```python
from build123d import *

# Parameters (mm, degrees)
SKETCH1_R            = 10
SKETCH1_R_2          = 5
BOSS_EXTRUDE1_DEPTH  = 10
SKETCH2_R            = 7
SKETCH2_R_2          = 5
BOSS_EXTRUDE2_DEPTH  = 3.5
SKETCH3_R            = 10
SKETCH3_R_2          = 5
BOSS_EXTRUDE3_DEPTH  = 10
SKETCH4_R            = 7
SKETCH4_R_2          = 5
BOSS_EXTRUDE4_DEPTH  = 3.5
SKETCH5_R            = 10
SKETCH5_R_2          = 5
BOSS_EXTRUDE5_DEPTH  = 10
SKETCH6_R            = 7
SKETCH6_R_2          = 5
BOSS_EXTRUDE6_DEPTH  = 3.5
SKETCH7_R            = 10
SKETCH7_R_2          = 5
BOSS_EXTRUDE7_DEPTH  = 10
SKETCH8_R            = 7
SKETCH8_R_2          = 5
BOSS_EXTRUDE8_DEPTH  = 3.5
SKETCH9_R            = 10
SKETCH9_R_2          = 5
BOSS_EXTRUDE9_DEPTH  = 10
SKETCH10_R           = 7
SKETCH10_R_2         = 5
BOSS_EXTRUDE10_DEPTH = 3.5
SKETCH11_R           = 10
SKETCH11_R_2         = 5
BOSS_EXTRUDE11_DEPTH = 10


with BuildPart() as part:
    # Sketch1 → Boss-Extrude1 (new body)
    with BuildSketch(Plane(origin=(0, 0, 0), x_dir=(1, 0, 0), z_dir=(0, 1, 0))):
        with Locations(Location((0, 0, 0), (0, 0, 270))):
            Circle(SKETCH1_R)
        with Locations(Location((0, 0, 0), (0, 0, 270))):
            Circle(SKETCH1_R_2, mode=Mode.SUBTRACT)
    extrude(amount=BOSS_EXTRUDE1_DEPTH)

    # Sketch2 → Boss-Extrude2 (add)
    with BuildSketch(Plane(origin=(0, 10, 0), x_dir=(1, 0, 0), z_dir=(0, 1, 0))):
        with Locations(Location((0, 0, 0), (0, 0, 270))):
            Circle(SKETCH2_R)
        with Locations(Location((0, 0, 0), (0, 0, 270))):
            Circle(SKETCH2_R_2, mode=Mode.SUBTRACT)
    extrude(amount=BOSS_EXTRUDE2_DEPTH)

    # Sketch3 → Boss-Extrude3 (add)
    with BuildSketch(Plane(origin=(0, 13.5, 0), x_dir=(1, 0, 0), z_dir=(0, 1, 0))):
        with Locations(Location((0, 0, 0), (0, 0, 270))):
            Circle(SKETCH3_R)
        with Locations(Location((0, 0, 0), (0, 0, 270))):
            Circle(SKETCH3_R_2, mode=Mode.SUBTRACT)
    extrude(amount=BOSS_EXTRUDE3_DEPTH)

    # Sketch4 → Boss-Extrude4 (add)
    with BuildSketch(Plane(origin=(0, 23.5, 0), x_dir=(1, 0, 0), z_dir=(0, 1, 0))):
        with Locations(Location((0, 0, 0), (0, 0, 270))):
            Circle(SKETCH4_R)
        with Locations(Location((0, 0, 0), (0, 0, 270))):
            Circle(SKETCH4_R_2, mode=Mode.SUBTRACT)
    extrude(amount=BOSS_EXTRUDE4_DEPTH)

    # Sketch5 → Boss-Extrude5 (add)
    with BuildSketch(Plane(origin=(0, 27, 0), x_dir=(1, 0, 0), z_dir=(0, 1, 0))):
        with Locations(Location((0, 0, 0), (0, 0, 270))):
            Circle(SKETCH5_R)
        with Locations(Location((0, 0, 0), (0, 0, 270))):
            Circle(SKETCH5_R_2, mode=Mode.SUBTRACT)
    extrude(amount=BOSS_EXTRUDE5_DEPTH)

    # Sketch6 → Boss-Extrude6 (add)
    with BuildSketch(Plane(origin=(0, 37, 0), x_dir=(1, 0, 0), z_dir=(0, 1, 0))):
        with Locations(Location((0, 0, 0), (0, 0, 270))):
            Circle(SKETCH6_R)
        with Locations(Location((0, 0, 0), (0, 0, 270))):
            Circle(SKETCH6_R_2, mode=Mode.SUBTRACT)
    extrude(amount=BOSS_EXTRUDE6_DEPTH)

    # Sketch7 → Boss-Extrude7 (add)
    with BuildSketch(Plane(origin=(0, 40.5, 0), x_dir=(1, 0, 0), z_dir=(0, 1, 0))):
        with Locations(Location((0, 0, 0), (0, 0, 270))):
            Circle(SKETCH7_R)
        with Locations(Location((0, 0, 0), (0, 0, 270))):
            Circle(SKETCH7_R_2, mode=Mode.SUBTRACT)
    extrude(amount=BOSS_EXTRUDE7_DEPTH)

    # Sketch8 → Boss-Extrude8 (add)
    with BuildSketch(Plane(origin=(0, 50.5, 0), x_dir=(1, 0, 0), z_dir=(0, 1, 0))):
        with Locations(Location((0, 0, 0), (0, 0, 270))):
            Circle(SKETCH8_R)
        with Locations(Location((0, 0, 0), (0, 0, 270))):
            Circle(SKETCH8_R_2, mode=Mode.SUBTRACT)
    extrude(amount=BOSS_EXTRUDE8_DEPTH)

    # Sketch9 → Boss-Extrude9 (add)
    with BuildSketch(Plane(origin=(0, 54, 0), x_dir=(1, 0, 0), z_dir=(0, 1, 0))):
        with Locations(Location((0, 0, 0), (0, 0, 270))):
            Circle(SKETCH9_R)
        with Locations(Location((0, 0, 0), (0, 0, 270))):
            Circle(SKETCH9_R_2, mode=Mode.SUBTRACT)
    extrude(amount=BOSS_EXTRUDE9_DEPTH)

    # Sketch10 → Boss-Extrude10 (add)
    with BuildSketch(Plane(origin=(0, 64, 0), x_dir=(1, 0, 0), z_dir=(0, 1, 0))):
        with Locations(Location((0, 0, 0), (0, 0, 270))):
            Circle(SKETCH10_R)
        with Locations(Location((0, 0, 0), (0, 0, 270))):
            Circle(SKETCH10_R_2, mode=Mode.SUBTRACT)
    extrude(amount=BOSS_EXTRUDE10_DEPTH)

    # Sketch11 → Boss-Extrude11 (add)
    with BuildSketch(Plane(origin=(0, 67.5, 0), x_dir=(1, 0, 0), z_dir=(0, 1, 0))):
        with Locations(Location((0, 0, 0), (0, 0, 270))):
            Circle(SKETCH11_R)
        with Locations(Location((0, 0, 0), (0, 0, 270))):
            Circle(SKETCH11_R_2, mode=Mode.SUBTRACT)
    extrude(amount=BOSS_EXTRUDE11_DEPTH)


solid = part.part
```
Build history of the part. All positions in model axes, mm. A direction names the side the tool comes from. Give positions to 0.01 mm unless a question says otherwise; leave off trailing zeros. Loops run counter-clockwise (first coordinate to the right, second up) from the corner with the lowest first, then second, coordinate; pieces in that order, holes last. Notation, with made-up numbers: (-32.75, 89.5) -> (16.25, 89.5) arc R16 cw to (16.25, 102.5) -> close; hole circle Ø8 at (76, 41). An arc over 180 degrees is marked (long way). One line per question, with ' | ' between items.
Q1. Tool access for faces 5 (the cylindrical face through (-9.76, 72.43, -2.17)), 6 (the flat face through (7, 50.5, 2)): list every direction of +Z, -Z, +X, -X, +Y, -Y with a clear straight run to the whole face (end or side of a thin tool).
Filled sheet:
face 5: +Y, -Y | face 6: none
Q2. Cut at B-B, the plane y = 21. Write the cut outline in (x, z), plus the area to 3 significant figures.
Filled sheet:
outline: circle Ø20 at (0, 0); hole circle Ø10 at (0, 0) | area: 236 mm²
Q3. Drill centre lines: line 1 along Y through (x, z) = (6, -5.5); line 2 along X through (y, z) = (52.5, 0); line 3 along X through (y, z) = (32, 0). Where is each one in solid material? Low to high. Write a range as [from, to].
Filled sheet:
line 1: y = [0, 10], [13.5, 23.5], [27, 37], [40.5, 50.5], [54, 64], [67.5, 77.5] | line 2: x = [-7, -5], [5, 7] | line 3: x = [-10, -5], [5, 10]
Q4. Cut at C-C, the plane y = 51.5. Write the cut outline in (x, z), plus the area to 3 significant figures.
Filled sheet:
outline: circle Ø14 at (0, 0); hole circle Ø10 at (0, 0) | area: 75.4 mm²
Q5. Pull direction Y, two halves, no side cores. Call faces 1 (the flat face through (5, 0, 2)), 2 (the cylindrical face through (-9.76, 18.43, -2.17)), 3 (the flat face through (5, 77.5, 2)), 4 (the cylindrical face through (-6.834, 52.226, -1.517)): pulls with the +Y half, pulls with the -Y half, needs draft (parallel to the pull), parting line crosses it, or undercut.
Filled sheet:
face 1: pulls with the -Y half | face 2: needs draft | face 3: pulls with the +Y half | face 4: undercut
Q6. Cut at A-A, the plane z = 8. Write the cut outline in (x, y), plus the area to 3 significant figures.
Filled sheet:
outline: (-6, 0) -> (6, 0) -> (6, 10) -> (-6, 10) -> close; (-6, 13.5) -> (6, 13.5) -> (6, 23.5) -> (-6, 23.5) -> close; (-6, 27) -> (6, 27) -> (6, 37) -> (-6, 37) -> close; (-6, 40.5) -> (6, 40.5) -> (6, 50.5) -> (-6, 50.5) -> close; (-6, 54) -> (6, 54) -> (6, 64) -> (-6, 64) -> close; (-6, 67.5) -> (6, 67.5) -> (6, 77.5) -> (-6, 77.5) -> close | area: 720 mm²
Q7. Drop flat-ended pins along their axis: pin 1 (4 mm diameter, centred on x = 1, z = 2, fed in from -Y) (1 decimal); pin 2 (5 mm diameter, centred on y = 54, z = 5, fed in from +X); pin 3 (4 mm diameter, centred on y = 45, z = -5, fed in from -X); pin 4 (6 mm diameter, centred on x = 7, y = 34, fed in from -Z). Give the stop position or say it passes through.
Filled sheet:
pin 1: passes through | pin 2: stops at x = 9.68 | pin 3: stops at x = -9.54 | pin 4: stops at z = -9.17
